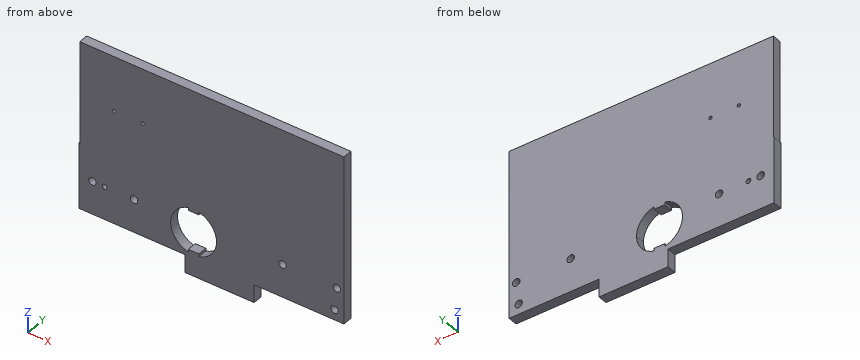
```python
from build123d import *

# Parameters (mm, degrees)
SKETCH1_R            = 3.96875
SKETCH1_R_2          = 2.55
SKETCH1_R_3          = 27.5336
BOSS_EXTRUDE7_DEPTH  = 10
SKETCH2_W            = 279.4
SKETCH2_H            = 10
BOSS_EXTRUDE8_DEPTH  = 108
CUT_EXTRUDE2_DEPTH   = 301.273208928
SKETCH3_7_R          = 1.7526
CUT_EXTRUDE3_DEPTH   = 35
SKETCH3_8_R          = 1.7526
CUT_EXTRUDE4_DEPTH   = 32
SKETCH2_3_W          = 279.4
SKETCH2_3_H          = 10
BOSS_EXTRUDE9_DEPTH  = 10
SKETCH10_W           = 73
SKETCH10_H           = 10
BOSS_EXTRUDE11_DEPTH = 19


with BuildPart() as part:
    # Sketch1 → Boss-Extrude7 (new body)
    with BuildSketch(Plane(origin=(0, 0, 0), x_dir=(1, 0, 0), z_dir=(0, 1, 0))):
        with BuildLine():
            Line((0, 70), (0, 0))
            Line((0, 0), (178.818297442, 0))
            ThreePointArc((178.818297442, 0), (164.66, 35), (178.818297442, 70))
            Line((178.818297442, 70), (0, 70))
        make_face()
        with Locations(Location((14, 35, 0), (0, 0, 270))):
            Circle(SKETCH1_R, mode=Mode.SUBTRACT)
        with Locations(Location((27, 35, 0), (0, 0, 270))):
            Circle(SKETCH1_R_2, mode=Mode.SUBTRACT)
        with Locations((58, 35)):
            Circle(SKETCH1_R_3, mode=Mode.SUBTRACT)
        with BuildLine():
            ThreePointArc((265.34, 35), (261.666382476, 16.122385039), (251.181702558, 0))
            Line((251.181702558, 0), (280, 0))
            Line((280, 0), (280, 70))
            Line((280, 70), (251.181702558, 70))
            ThreePointArc((251.181702558, 70), (261.666382476, 53.877614961), (265.34, 35))
        make_face()
        with Locations(Location((272.5, 35, 0), (0, 0, 270))):
            Circle(SKETCH1_R, mode=Mode.SUBTRACT)
        with Locations(Location((270, 59, 0), (0, 0, 270))):
            Circle(SKETCH1_R, mode=Mode.SUBTRACT)
        with BuildLine():
            ThreePointArc((178.818297442, 70), (164.66, 35), (178.818297442, 0))
            Line((178.818297442, 0), (251.181702558, 0))
            ThreePointArc((251.181702558, 0), (261.666382476, 16.122385039), (265.34, 35))
            ThreePointArc((265.34, 35), (261.666382476, 53.877614961), (251.181702558, 70))
            Line((251.181702558, 70), (178.818297442, 70))
        make_face()
        with Locations((215, 35)):
            Circle(SKETCH1_R_3, mode=Mode.SUBTRACT)
        with Locations((215, 35)):
            Circle(SKETCH1_R_3)
        with Locations(Location((215, 35, 0), (0, 0, 270))):
            Circle(SKETCH1_R, mode=Mode.SUBTRACT)
        with Locations((58, 35)):
            Circle(SKETCH1_R_3)
        with Locations(Location((58, 35, 0), (0, 0, 270))):
            Circle(SKETCH1_R, mode=Mode.SUBTRACT)
    extrude(amount=BOSS_EXTRUDE7_DEPTH)

    # Sketch2 → Boss-Extrude8 (add)
    with BuildSketch(Plane.XY):
        with Locations((140.3, 5)):
            Rectangle(SKETCH2_W, SKETCH2_H)
    extrude(amount=BOSS_EXTRUDE8_DEPTH)

    # Sketch3 → Cut-Extrude2 (cut, through all)
    with BuildSketch(Plane(origin=(0, 10, 0), x_dir=(1, 0, 0), z_dir=(0, 1, 0))):
        with BuildLine():
            Line((115.360720333, 62.78), (115.360720333, 65.616031098))
            ThreePointArc((115.360720333, 65.616031098), (96.72, 42), (115.360720333, 18.383968902))
            Line((115.360720333, 18.383968902), (115.360720333, 21.22))
            Line((115.360720333, 21.22), (126.639279667, 21.22))
            Line((126.639279667, 21.22), (126.639279667, 18.383968902))
            ThreePointArc((126.639279667, 18.383968902), (140.058332959, 26.956784092), (145.28, 42))
            ThreePointArc((145.28, 42), (140.058332959, 57.043215908), (126.639279667, 65.616031098))
            Line((126.639279667, 65.616031098), (126.639279667, 62.78))
            Line((126.639279667, 62.78), (115.360720333, 62.78))
        make_face()
    extrude(amount=-CUT_EXTRUDE2_DEPTH, mode=Mode.SUBTRACT)

    # Sketch3_7 → Cut-Extrude3 (cut)
    with BuildSketch(Plane(origin=(0, 10, 0), x_dir=(1, 0, 0), z_dir=(0, 1, 0))):
        with Locations(Location((37.1, -50, 0), (0, 0, 270))):
            Circle(SKETCH3_7_R)
    extrude(amount=-CUT_EXTRUDE3_DEPTH, mode=Mode.SUBTRACT)

    # Sketch3_8 → Cut-Extrude4 (cut)
    with BuildSketch(Plane(origin=(0, 10, 0), x_dir=(1, 0, 0), z_dir=(0, 1, 0))):
        with Locations(Location((67.1, -50, 0), (0, 0, 270))):
            Circle(SKETCH3_8_R)
    extrude(amount=-CUT_EXTRUDE4_DEPTH, mode=Mode.SUBTRACT)

    # Sketch2_3 → Boss-Extrude9 (add)
    with BuildSketch(Plane.XY):
        with Locations((140.3, 5)):
            Rectangle(SKETCH2_3_W, SKETCH2_3_H)
    extrude(amount=BOSS_EXTRUDE9_DEPTH)

    # Sketch10 → Boss-Extrude11 (add)
    with BuildSketch(Plane(origin=(0, 0, -70), x_dir=(-1, 0, 0), z_dir=(0, 0, -1))):
        with Locations((-148.5, 5)):
            Rectangle(SKETCH10_W, SKETCH10_H)
    extrude(amount=BOSS_EXTRUDE11_DEPTH)


solid = part.part
```
For this review, take the finished solid that the model builds, in its own axes (mm). Round coordinates to 2 decimals unless told otherwise and drop trailing zeros. Write each loop counter-clockwise with the first axis right and the second up, starting at its lowest first coordinate (ties: lowest second). Pieces come first, ordered by that corner, then holes. Notation, with made-up numbers: (87, 30.5) - (137, 30.5) arc R21 cw to (137, 60.5) - close; hole circle Ø7 at (79, 11.5). An arc over 180 degrees is marked (long way). Answer as a JSON object with one key per item and string values.
1. We need section C-C on z = -59. Give the boundary of the cut face in (x, y).
Response values:
{"outline": "(0, 0) - (103.66, 0) - (103.66, 10) - (0, 10) - close; (138.34, 0) - (266.03, 0) - (266.03, 10) - (138.34, 10) - close; (273.97, 0) - (280, 0) - (280, 10) - (273.97, 10) - close"}
2. To check wall thickness, follow line 1 along X through (y, z) = (5, 50); line 2 along Z through (x, y) = (272.5, 7.75); line 3 along Z through (x, y) = (67, 9). State the ranges of each line that lie inside material, in increasing order.
Response values:
{"line 1": "x = 0.6 to 35.35, 38.85 to 65.35, 68.85 to 280", "line 2": "z = -70 to -62.08, -55.92 to -38.97, -31.03 to 108", "line 3": "z = -70 to 48.25, 51.75 to 108"}
3. We need section A-A on y = 2.5. Count the separate pieces of the cut face and the enclosed holes in it, then the cut area to 3 significant figures.
Response values:
{"separate pieces": "1", "enclosed holes": "9", "area": "49,100 mm2"}
4. For pin 1 Ø3 at (x, y) = (81, 9) entering from -Z; pin 2 Ø3 at (y, z) = (5, 33) entering from -X; pin 3 Ø5 at (y, z) = (5, -80) entering from +X, all flat-tipped, find the tip position at first contact; note any pin that passes through.
Response values:
{"pin 1": "stops at z = -70", "pin 2": "stops at x = 0.6", "pin 3": "stops at x = 185"}
5. We need section D-D on x = 74. Give the boundary of the cut face in (y, z).
Response values:
{"outline": "(0, -70) - (10, -70) - (10, 108) - (0, 108) - close"}
6. We need section B-B on x = 14. Give the boundary of the cut face in (y, z), then the cut area to 3 significant figures.
Response values:
{"outline": "(0, -70) - (10, -70) - (10, -38.97) - (0, -38.97) - close; (0, -31.03) - (10, -31.03) - (10, 108) - (0, 108) - close", "area": "1,700 mm2"}
